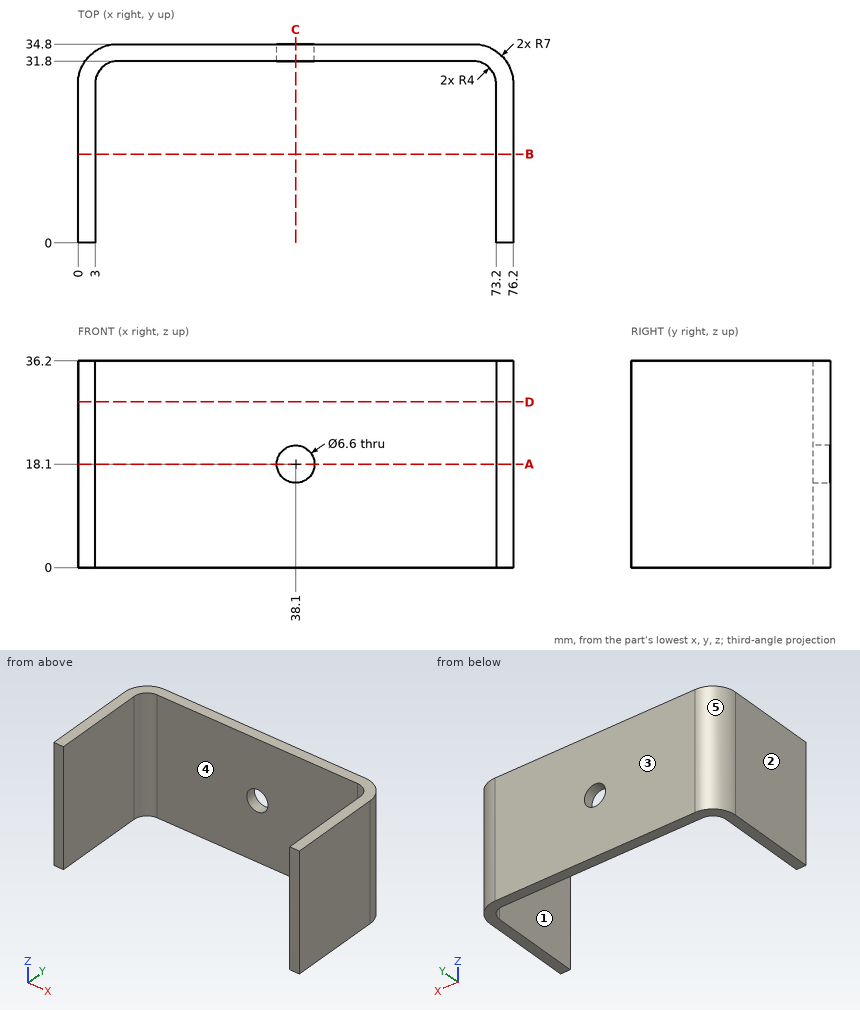
Can you work these out from the drawing? Everything is in mm from the part's minimum corner. A direction names the side the tool comes from. Give positions to 0.01 mm unless a question says otherwise; leave off trailing zeros. Order: outer loops, then holes, each group sorted by start corner. A loop starts at its lowest first (then second) coordinate and runs counter-clockwise, first axis right, second up.
1. Suppose I cut it at A-A (z = 18.1). List the corners of the cut face in (x, y) for me, plus the area to 3 significant figures.
2. Suppose I cut it at B-B (y = 15.5). List the corners of the cut face in (x, z) for me.
3. Suppose I cut it at D-D (z = 29). List the corners of the cut face in (x, y) for me, plus the area to 3 significant figures.
4. For the marked faces 4 and 5, which set-ups out of +Z, -Z, +X, -X, +Y, -Y let a thin tool reach every point of the face, with its end or its side?
5. Will this pin go through, and if not, where does the flat tip stop? P1, Ø1, axis at x = 14.5, z = 12, coming from the -Y side.
6. I need wall thicknesses on L1, parallel to X at y = 4, z = 5; L2, parallel to Y at x = 17, z = 23.5; L3, parallel to X at y = 32.4, z = 18.1. Which ranges of each line are inside material? Lowest first, please.
7. We'd pull the mould along X, two halves only. Please class the marked faces 1, 2 and 3: pulls with the +X half, pulls with the -X half, needs draft (parallel to the pull), parting line crosses it, or undercut.
8. Suppose I cut it at C-C (x = 38.1). List the corners of the cut face in (y, z) for me, plus the area to 3 significant figures.
Solved:
1. outline: (0, 0) - (3, 0) - (3, 27.8) arc R4 cw to (7, 31.8) - (34.8, 31.8) - (34.8, 34.8) - (7, 34.8) arc R7 ccw to (0, 27.8) - close; (41.4, 31.8) - (69.2, 31.8) arc R4 cw to (73.2, 27.8) - (73.2, 0) - (76.2, 0) - (76.2, 27.8) arc R7 ccw to (69.2, 34.8) - (41.4, 34.8) - close
1. area: 385 mm2
2. outline: (0, 0) - (3, 0) - (3, 36.2) - (0, 36.2) - close; (73.2, 0) - (76.2, 0) - (76.2, 36.2) - (73.2, 36.2) - close
3. outline: (0, 0) - (3, 0) - (3, 27.8) arc R4 cw to (7, 31.8) - (69.2, 31.8) arc R4 cw to (73.2, 27.8) - (73.2, 0) - (76.2, 0) - (76.2, 27.8) arc R7 ccw to (69.2, 34.8) - (7, 34.8) arc R7 ccw to (0, 27.8) - close
3. area: 405 mm2
4. face 4: +Z, -Z, -Y
4. face 5: +Z, -Z, -X, +Y
5. P1: stops at y = 31.8
6. L1: x = 0 to 3, 73.2 to 76.2
6. L2: y = 31.8 to 34.8
6. L3: x = 1.72 to 34.8, 41.4 to 74.48
7. face 1: undercut
7. face 2: pulls with the -X half
7. face 3: needs draft
8. outline: (31.8, 0) - (34.8, 0) - (34.8, 14.8) - (31.8, 14.8) - close; (31.8, 21.4) - (34.8, 21.4) - (34.8, 36.2) - (31.8, 36.2) - close
8. area: 88.8 mm2
